Can you work these out from the model? Positions are in its coordinate system, mm. Coordinates: 2 decimals unless noted, no trailing zeros. Order: outer loops, then holes, each group sorted by start corner. A loop starts at its lowest first (then second) coordinate and runs counter-clockwise, first axis right, second up. Notation, with made-up numbers: (81, 77) -> (137, 77) arc R18 cw to (137, 95) -> close; hole circle Ø5 at (21, -21.5). An arc over 180 degrees is marked (long way). Answer as CSV lines item,"result".
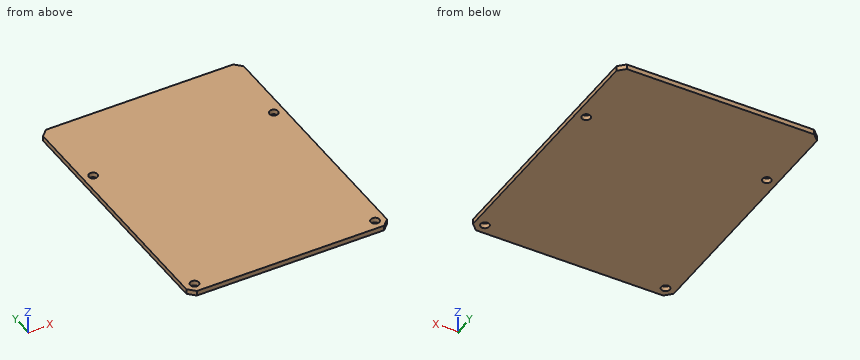
from build123d import *

# Parameters (mm, degrees)
SKETCH_1_W          = 60
SKETCH_1_H          = 79
EXTRUDE_1_DEPTH     = 1.5
CHAMFER_1_SIZE      = 2
HOLE_WIZARD_M2_51_D = 2.55


with BuildPart() as part:
    # Эскиз1 → Бобышка-Вытянуть1 (new body)
    with BuildSketch(Plane.XY):
        Rectangle(SKETCH_1_W, SKETCH_1_H)
    extrude(amount=EXTRUDE_1_DEPTH)

    # Фаска1
    chamfer_1_edges = [part.edges().sort_by_distance(p)[0] for p in [
        (30, -39.5, 0.75),
        (-30, -39.5, 0.75),
        (-30, 39.5, 0.75),
        (30, 39.5, 0.75),
    ]]
    chamfer(chamfer_1_edges, length=CHAMFER_1_SIZE)

    # Сверло под метчик  спиральное M2.51 (through all)
    with Locations(Plane.XY.offset(1.5)):
        with Locations((-27, 16.5), (27, 16.5), (27, -36.5), (-27, -36.5)):
            Hole(HOLE_WIZARD_M2_51_D / 2)


solid = part.part
Q1. For P1, Ø8, axis at x = -1.5, y = 12.5, coming from the -Z side, with a flat end and sliding along its axis, tell me the tip position at first contact or that it passes through.
Solution:
P1,"z = 0"
Q2. If I drill on line 1 (Y direction, x = -27, z = 0.3) (3 decimals); line 2 (X direction, y = 15.5, z = 0.3); line 3 (X direction, y = -36, z = 1.3), over which ranges is the centre line in solid material (lowest first)?
Solution:
line 1,"-39.5 to -37.775, -35.225 to 15.225, 17.775 to 39.5"
line 2,"-30 to -27.79, -26.21 to 26.21, 27.79 to 30"
line 3,"-30 to -28.17, -25.83 to 25.83, 28.17 to 30"
Q3. Imagine slicing it at A-A (x = 27). List the corners of the cut face in (y, z) for me (3 decimals), and give its area (3 significant figures).
Solution:
outline,"(-39.5, 0) -> (-37.775, 0) -> (-37.775, 1.5) -> (-39.5, 1.5) -> close; (-35.225, 0) -> (15.225, 0) -> (15.225, 1.5) -> (-35.225, 1.5) -> close; (17.775, 0) -> (39.5, 0) -> (39.5, 1.5) -> (17.775, 1.5) -> close"
area,"111 mm2"
Q4. Imagine slicing it at B-B (y = 16.5). List the corners of the cut face in (x, z) for me (3 decimals), and give its area (4 significant figures).
Solution:
outline,"(-30, 0) -> (-28.275, 0) -> (-28.275, 1.5) -> (-30, 1.5) -> close; (-25.725, 0) -> (25.725, 0) -> (25.725, 1.5) -> (-25.725, 1.5) -> close; (28.275, 0) -> (30, 0) -> (30, 1.5) -> (28.275, 1.5) -> close"
area,"82.35 mm2"
